```python
from build123d import *

# Parameters (mm, degrees)
F0_W          = 1.5875
F0_H          = 38.1
F1_DEPTH      = 63.5
F2_W          = 1.78622
F2_H          = 24.92076
F3_DEPTH      = 3.175
F5_W          = 21.454677
F5_H          = 27.739912
F6_DEPTH      = 25.4
F6_DEPTH_BACK = 25.4
F7_DEPTH      = 25.4


with BuildPart() as f1:
    # F0 (on Front) → F1 (new body)
    with BuildSketch(Plane.XZ):
        Rectangle(F0_W, F0_H)
    extrude(amount=F1_DEPTH)

    # F2 (on face) → F3 (join)
    with BuildSketch(Plane.YZ.offset(0.79375)):
        with Locations((-31.75, 0)):
            Rectangle(F2_W, F2_H)
    extrude(amount=F3_DEPTH)

    # F5 (on face) → F6 (cut, two sides)
    with BuildSketch(Plane.YZ.offset(0.79375)) as f6_sk:
        with Locations((-18.722475, 0)):
            Rectangle(F5_W, F5_H)
    extrude(amount=-F6_DEPTH, mode=Mode.SUBTRACT)
    extrude(f6_sk.sketch, amount=-F6_DEPTH_BACK, mode=Mode.SUBTRACT)

    # F4 (on face) → F7 (join)
    with BuildSketch(Plane.XY.offset(12.46038)):
        Polygon((2.38125, -30.85689), (3.96875, -30.85689), (-1.625961, -9.949325), (-2.755997, -10.251714), (-0.909572, -21.768624), align=None)
    extrude(amount=-F7_DEPTH)


solid = f1.part
```
The model under review builds one solid part; all positions refer to its coordinate system, in mm. A direction names the side the tool comes from. Round coordinates to 2 decimals unless told otherwise and drop trailing zeros. Order: outer loops, then holes, each group sorted by start corner. A loop starts at its lowest first (then second) coordinate and runs counter-clockwise, first axis right, second up. Notation, with made-up numbers: (-32, 34.5) -> (20, 34.5) arc R25 ccw to (20, 66.5) -> close; hole circle Ø6 at (30, 68.5). An arc over 180 degrees is marked (long way). Use a Markdown table: item, result.
Q1. Clearance check with flat-ended pins moving along their axes: P1, Ø6, axis at y = -41, z = 15, coming from the -X side; P2, Ø0.5, axis at x = 3, z = -12.5, coming from the -Y side; P3, Ø4, axis at x = 2, y = -33, coming from the +Z side; P4, Ø2, axis at x = 2.5, y = -31.5, coming from the -Z side. State where each tip first meets the part, or that it passes through.
Values:
| item | result |
|---|---|
| P1 | stops at x = -0.79 |
| P2 | stops at y = -32.64 |
| P3 | stops at z = 19.05 |
| P4 | stops at z = -12.94 |
Q2. Mouldability with a two-part tool opening along Z and no side actions: class faces 1 (the flat face through (0, -29.45, 0)), 2 (the flat face through (0, -63.5, 0)), 3 (the flat face through (2, -32, -12.46)) as +Z half, -Z half, draft (parallel to the pull), parting line (faces both ways), or undercut.
Values:
| item | result |
|---|---|
| face 1 | undercut |
| face 2 | draft |
| face 3 | -Z half |
Q3. We need section D-D on z = -14.5. Write out the cut boundary in (x, y), then the cut area to 3 significant figures.
Values:
| item | result |
|---|---|
| outline | (-0.79, -63.5) -> (0.79, -63.5) -> (0.79, 0) -> (-0.79, 0) -> close |
| area | 101 mm^2 |
Q4. Tool access review of faces 4 (the flat face through (0, -19, -13.87)), 5 (the flat face through (1.21, -20.55, -0.06)), 6 (the flat face through (2, -32.643, 0)): name each direction out of +Z, -Z, +X, -X, +Y, -Y from which nothing blocks a thin tool from reaching the whole face with its end or side.
Values:
| item | result |
|---|---|
| face 4 | +X, -X |
| face 5 | +X |
| face 6 | +Z, -Z, +X, -Y |
Q5. We need section A-A on z = 7. Write out the cut boundary in (x, y).
Values:
| item | result |
|---|---|
| outline | (-2.76, -10.25) -> (-0.91, -21.77) -> (2.38, -30.86) -> (0.79, -30.86) -> (0.79, -29.45) -> (-0.79, -29.45) -> (-0.79, -63.5) -> (0.79, -63.5) -> (0.79, -32.64) -> (3.97, -32.64) -> (3.97, -30.86) -> (-1.63, -9.95) -> close; (-0.79, -8) -> (0.79, -8) -> (0.79, 0) -> (-0.79, 0) -> close |
Q6. We need section C-C on x = 1.75. Write out the cut boundary in (y, z), then the cut area to 3 significant figures.
Values:
| item | result |
|---|---|
| outline | (-32.64, -12.46) -> (-30.86, -12.46) -> (-30.86, 12.46) -> (-32.64, 12.46) -> close; (-29.11, -12.94) -> (-22.57, -12.94) -> (-22.57, 12.46) -> (-29.11, 12.46) -> close |
| area | 211 mm^2 |
Q7. For line 1 (Z direction, x = 0, y = -14); line 2 (X direction, y = -15.5, z = 15); line 3 (Z direction, x = -1.25, y = -15.5), list the stretches that pass through material, from the lowest coordinate up.
Values:
| item | result |
|---|---|
| line 1 | z = -19.05 to -13.87, 13.87 to 19.05 |
| line 2 | x = -0.79 to 0.79 |
| line 3 | z = -12.94 to 12.46 |
Q8. We need section B-B on y = -21. Write out the cut boundary in (x, z).
Values:
| item | result |
|---|---|
| outline | (-1.03, -12.94) -> (1.33, -12.94) -> (1.33, 12.46) -> (-1.03, 12.46) -> close; (-0.79, -19.05) -> (0.79, -19.05) -> (0.79, -13.87) -> (-0.79, -13.87) -> close; (-0.79, 13.87) -> (0.79, 13.87) -> (0.79, 19.05) -> (-0.79, 19.05) -> close |
